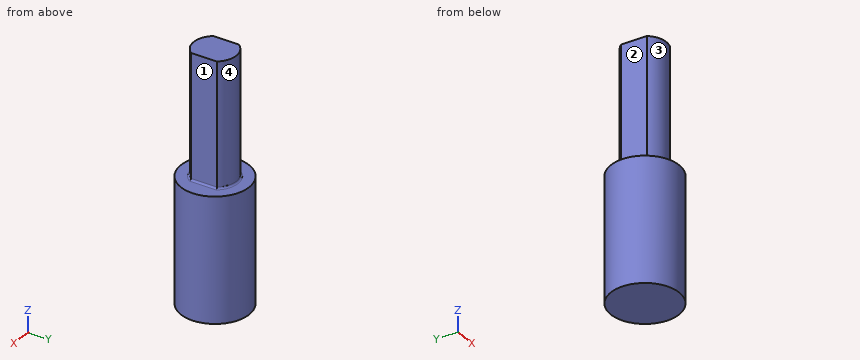
from build123d import *

# Parameters (mm, degrees)
ESQUISSE1_R        = 19.25
ESQUISSE1_R_2      = 12
ESQUISSE1_W        = 19
ESQUISSE1_H        = 14.662878298
BOSS_EXTRU_1_DEPTH = 70
ESQUISSE1_4_W      = 19
ESQUISSE1_4_H      = 14.662878298
BOSS_EXTRU_2_DEPTH = 70
CONG_1_R           = 1


with BuildPart() as part:
    # Esquisse1 → Boss.-Extru.1 (new body)
    with BuildSketch(Plane.XY):
        Circle(ESQUISSE1_R)
        Circle(ESQUISSE1_R_2, mode=Mode.SUBTRACT)
        Rectangle(ESQUISSE1_W, ESQUISSE1_H)
        with BuildLine():
            Line((9.5, 7.331439149), (9.5, -7.331439149))
            ThreePointArc((9.5, -7.331439149), (11.357816692, -3.872983346), (12, 0))
            ThreePointArc((12, 0), (11.357816692, 3.872983346), (9.5, 7.331439149))
        make_face()
        with BuildLine():
            Line((9.5, -7.331439149), (-9.5, -7.331439149))
            ThreePointArc((-9.5, -7.331439149), (0, -12), (9.5, -7.331439149))
        make_face()
        with BuildLine():
            ThreePointArc((-9.5, 7.331439149), (-12, 0), (-9.5, -7.331439149))
            Line((-9.5, -7.331439149), (-9.5, 7.331439149))
        make_face()
        with BuildLine():
            ThreePointArc((9.5, 7.331439149), (0, 12), (-9.5, 7.331439149))
            Line((-9.5, 7.331439149), (9.5, 7.331439149))
        make_face()
    extrude(amount=-BOSS_EXTRU_1_DEPTH)

    # Esquisse1_4 → Boss.-Extru.2 (add)
    with BuildSketch(Plane.XY):
        with BuildLine():
            ThreePointArc((9.5, 7.331439149), (0, 12), (-9.5, 7.331439149))
            Line((-9.5, 7.331439149), (9.5, 7.331439149))
        make_face()
        Rectangle(ESQUISSE1_4_W, ESQUISSE1_4_H)
        with BuildLine():
            Line((9.5, -7.331439149), (-9.5, -7.331439149))
            ThreePointArc((-9.5, -7.331439149), (0, -12), (9.5, -7.331439149))
        make_face()
    extrude(amount=BOSS_EXTRU_2_DEPTH)

    # Cong_1
    cong_1_edges = [part.edges().sort_by_distance(p)[0] for p in [
        (0, 12, 0),
        (0, -12, 0),
        (9.5, 0, 0),
        (-9.5, 0, 0),
    ]]
    fillet(cong_1_edges, radius=CONG_1_R)


solid = part.part
Work out the finished part from the listing and answer in its coordinate system (mm). Face numbers are marked on the shaded views. A direction names the side the tool comes from. Round coordinates to 2 decimals unless told otherwise and drop trailing zeros. Write each loop counter-clockwise with the first axis right and the second up, starting at its lowest first coordinate (ties: lowest second). Pieces come first, ordered by that corner, then holes. Notation, with made-up numbers: (-33, 16.5) -> (25, 16.5) arc R13 cw to (25, 39.5) -> close; hole circle Ø3 at (66.25, 48). An arc over 180 degrees is marked (long way). Answer as CSV lines item,"result". Start each with the question number.
(1) The part is cut by section C-C, the plane z = 39. Give the vertices of the cut face in (x, y), then the cut area to 3 significant figures.
(2) The part is cut by section D-D, the plane z = -20. Give the vertices of the cut face in (x, y).
(3) The part is cut by section A-A, the plane x = 0. Give the vertices of the cut face in (y, z), then the cut area to 3 significant figures.
(4) A tool of negligible diameter and unlimited length cuts with its end or side. For the marked faces 1, 2, 3 and 4, from which of +Z, -Z, +X, -X, +Y, -Y can it reach the whole face along a straight path? Write none if from no direction.
(5) Each of these flat-tipped pins is pushed along its axis until it touches: pin 1 (5 mm diameter, centred on y = -5.5, z = 9.5, fed in from +X); pin 2 (3 mm diameter, centred on x = 10.5, z = 9, fed in from -Y); pin 3 (4 mm diameter, centred on x = -13, y = -5, fed in from +Z). Where does it stop, or does it pass through?
(6) Find the intervals of material crossed by probe 1 along Y at (x, z) = (0, -24); probe 2 along Z at (x, y) = (-15, 9); probe 3 along X at (y, z) = (-9.5, 39.5), in increasing order.
(7) The part is cut by section B-B, the plane y = 0. Give the vertices of the cut face in (x, z), then the cut area to 3 significant figures.
Output values:
1,outline,"(-9.5, -7.33) arc R12 ccw to (9.5, -7.33) -> (9.5, 7.33) arc R12 ccw to (-9.5, 7.33) -> close"
1,area,"402 mm²"
2,outline,"circle Ø38.5 at (0, 0)"
3,outline,"(-19.25, -70) -> (19.25, -70) -> (19.25, 0) -> (13, 0) arc R1 cw to (12, 1) -> (12, 70) -> (-12, 70) -> (-12, 1) arc R1 cw to (-13, 0) -> (-19.25, 0) -> close"
3,area,"4,380 mm²"
4,face 1,"+Z, +X, +Y, -Y"
4,face 2,"+Z, -X, +Y, -Y"
4,face 3,"+Z, -Y"
4,face 4,"+Z, +Y"
5,pin 1,"stops at x = 9.5"
5,pin 2,"stops at y = -7.94"
5,pin 3,"stops at z = 0"
6,probe 1,"y = -19.25 to 19.25"
6,probe 2,"z = -70 to 0"
6,probe 3,"x = -7.33 to 7.33"
7,outline,"(-19.25, -70) -> (19.25, -70) -> (19.25, 0) -> (10.5, 0) arc R1 cw to (9.5, 1) -> (9.5, 70) -> (-9.5, 70) -> (-9.5, 1) arc R1 cw to (-10.5, 0) -> (-19.25, 0) -> close"
7,area,"4,030 mm²"
